Here's how the part is built. I have some questions about the finished solid (model axes, mm). A direction names the side the tool comes from. Give positions to 0.01 mm unless a question says otherwise; leave off trailing zeros. Order: outer loops, then holes, each group sorted by start corner. A loop starts at its lowest first (then second) coordinate and runs counter-clockwise, first axis right, second up.
from build123d import *


with BuildPart() as part:
    # Sketch1 → Revolve2 (revolve)
    with BuildSketch(Plane(origin=(0, 0, 0), x_dir=(0, 0, -1), z_dir=(1, 0, 0)), mode=Mode.PRIVATE) as revolve2_sk:
        Polygon((-3.366397964, 7), (2, 7), (2, 0), (0, 0), (-4.5, 7.794228634), (-3.82494608, 7.794228634), align=None)
        Polygon((1, 6.4), (1, 1.4), (0, 1.4), (-2.886751346, 6.4), align=None, mode=Mode.SUBTRACT)
    revolve(revolve2_sk.sketch.rotate(Axis((0, 0, -4), (0, 1, 0)), 180), axis=Axis((0, 0, -4), (0, 1, 0)))


solid = part.part
Q1. If we section it at D-D on x = -2.75: Give the number of separate pieces and of enclosed holes in the cut face, plus the area to 3 significant figures.
Filled sheet:
separate pieces: 1
enclosed holes: 2
area: 40.9 mm2
Q2. If we section it at C-C on y = 3.5: List the corners of the cut face in (x, z) for me.
Filled sheet:
outline: circle Ø12.04 at (0, -4); circle Ø6 at (0, -4); hole circle Ø10.42 at (0, -4); hole circle Ø4 at (0, -4)
Q3. For faces 1 (the face through (1, 6.4, -7)), 2 (the face through (4, 7.794, -11)), 3 (the face through (2, 7, -6)), which set-ups out of +Z, -Z, +X, -X, +Y, -Y let a thin tool reach every point of the face, with its end or its side?
Filled sheet:
face 1: none
face 2: +Z, -Z, +X, -X, +Y
face 3: +Y
Q4. If we section it at A-A on z = -4: List the corners of the cut face in (x, y) for me.
Filled sheet:
outline: (-8.5, 7.79) - (-4, 0) - (-2, 0) - (-2, 7) - (-7.37, 7) - (-7.82, 7.79) - close; (2, 0) - (4, 0) - (8.5, 7.79) - (7.82, 7.79) - (7.37, 7) - (2, 7) - close; hole (-6.89, 6.4) - (-4, 1.4) - (-3, 1.4) - (-3, 6.4) - close; hole (3, 1.4) - (4, 1.4) - (6.89, 6.4) - (3, 6.4) - close
Q5. If we section it at B-B on x = 0: List the corners of the cut face in (y, z) for me, plus the area to 3 significant figures.
Filled sheet:
outline: (0, -8) - (7.79, -12.5) - (7.79, -11.82) - (7, -11.37) - (7, -6) - (0, -6) - close; (0, -2) - (7, -2) - (7, 3.37) - (7.79, 3.82) - (7.79, 4.5) - (0, 0) - close; hole (1.4, -8) - (6.4, -10.89) - (6.4, -7) - (1.4, -7) - close; hole (1.4, -1) - (6.4, -1) - (6.4, 2.89) - (1.4, 0) - close
area: 32.9 mm2
Q6. Thinking about a two-plate mould opening in Z: for faces 4 (the face through (-2, 0, -3)), 5 (the face through (1.2, 3.5, -2.4)), 6 (the face through (1.831, 1.354, -8.417)), which applies, released by +Z, released by -Z, zero draft, split by the parting line, or undercut?
Filled sheet:
face 4: zero draft
face 5: undercut
face 6: split by the parting line
Q7. I'm going to push flat-ended pins straight in: P1, Ø4, axis at y = 2, z = -1, coming from the -X side; P2, Ø4, axis at y = 2, z = 0, coming from the +X side; P3, Ø2.5, axis at x = 0, z = -4, coming from the -Y side; P4, Ø4, axis at x = -2, z = -2, coming from the -Y side. Where does each tip first touch, or does it pass through?
Filled sheet:
P1: stops at x = -5.82
P2: stops at x = 5.4
P3: passes through
P4: stops at y = 0
Q8. I need wall thicknesses on L1, parallel to X at y = 3.5, z = -4; L2, parallel to Z at x = 1.25, y = 5; L3, parallel to Z at x = 1.5, y = 5.75. Which ranges of each line are inside material? Lowest first, please.
Filled sheet:
L1: x = -6.02 to -5.21, -3 to -2, 2 to 3, 5.21 to 6.02
L2: z = -10.77 to -9.95, -6.73 to -5.56, -2.44 to -1.27, 1.95 to 2.77
L3: z = -11.16 to -10.34, -6.6 to -5.32, -2.68 to -1.4, 2.34 to 3.16
